Autodesk Inventor part; units mm, degrees
ref_plane "YZ Plane" through (0, 0, 0) normal (1, 0, 0) x (0, 1, 0)
ref_plane "XZ Plane" through (0, 0, 0) normal (0, 1, 0) x (-1, 0, 0)
ref_plane "XY Plane" through (0, 0, 0) normal (0, 0, 1) x (1, 0, 0)
ref_plane "Work Plane1" through (32.4858, 0, 0) normal (0, 0, 1) x (1, 0, 0)
sketch "Sketch1" plane through (32.4858, 0, 0) normal (0, 0, 1) x (1, 0, 0)
  line L0 (-82.3611, -0.4) -> (-82.3611, 2.4)
  line L1 (-32.4858, 2) -> (-181.2976, 2)
  line L2 (-32.4858, 55) -> (-181.2976, 55)
  line L3 (-82.3611, 54.6) -> (-82.3611, 57.4)
  line L4 (-157.3611, 54.6) -> (-157.3611, 57.4)
  line L5 (-157.3611, -0.4) -> (-157.3611, 2.4)
  line L6 (-107.3611, -0.4) -> (-107.3611, 2.4)
  line L7 (-132.3611, -0.4) -> (-132.3611, 2.4)
  line L8 (-107.3611, 54.6) -> (-107.3611, 57.4)
  line L9 (-132.3611, 54.6) -> (-132.3611, 57.4)
  line L10 (-32.4858, 0) -> (-181.2976, 0)
  line L11 (-32.4858, 57) -> (-181.2976, 57)
  line L12 (-82.3611, 2) -> (-82.3611, 55) construction
  line L13 (-157.3611, 2) -> (-157.3611, 55) construction
  line L14 (-77.3611, 2) -> (-77.3611, 55)
  line L15 (-162.3611, 2) -> (-162.3611, 55)
  dimension "d0" = 5
  dimension "d1" = 5
ref_plane "Work Plane3" through (-129.8754, 2, 0) normal (1, 0, 0) x (0, 1, 0)
ref_plane "Work Plane2" through (1.0604, 0, 0) normal (0, 0, 1) x (-1, 0, 0)
sketch "Sketch2" plane through (-129.8754, 2, 0) normal (1, 0, 0) x (0, 1, 0)
  line L0 (0, 8.3309) -> (0, -17.2762)
  line L1 (53, 8.3309) -> (53, -17.2762)
  line L2 (53, -34) -> (55, -34)
  line L3 (53, -34) -> (55, -34)
  line L4 (-2, -34) -> (0, -34)
  line L5 (-2, -34) -> (0, -34)
  line L6 (53, -34) -> (0, -34) construction
  line L7 (53, -36) -> (0, -36)
  line L8 (0, 0) -> (53, 0) construction
  line L9 (0, 0) -> (0, -8) construction
  line L10 (53, 0) -> (53, -8) construction
  line L11 (47.871, -33) -> (5.129, -33)
  line L12 (53, -29) -> (0, -29) construction
  line L13 (53, 2) -> (0, 2)
  line L14 (47.871, -1) -> (5.129, -1)
  line L15 (53, -5) -> (0, -5) construction
  line L16 (5.129, -33) -> (26.5, -20.5)
  line L17 (32.4839, -17) -> (53, -5)
  line L18 (5.129, -1) -> (26.5, -13.5)
  line L19 (32.4839, -17) -> (53, -29)
  line L20 (0, -29) -> (20.5161, -17)
  line L21 (26.5, -13.5) -> (47.871, -1)
  line L22 (0, -5) -> (20.5161, -17)
  line L23 (26.5, -20.5) -> (47.871, -33)
  line L24 (53, 2) -> (53, -5)
  line L25 (0, 2) -> (0, -5)
  line L26 (0, -29) -> (0, -36)
  line L27 (53, -29) -> (53, -36)
  point P0 (-2, 0)
  dimension "d20" = 2
  dimension "d37" = 1
  dimension "d38" = 4
  dimension "d39" = 2
  dimension "d40" = 1
  dimension "d41" = 4
extrude "Extrusion2" add sketch "Sketch2" along normal blind 85
sketch "Sketch3" plane through (-129.8754, 55, -29) normal (0, 1, 0) x (1, 0, 0)
  line L0 (0, -12) -> (85, -12)
  point P0 (129.8754, -29)
sketch "Sketch4" plane through (-129.8754, 2, 0) normal (-1, 0, 0) x (0, 0, 1)
  line L0 (-13.5, 26.5) -> (-1, 47.871)
  line L1 (-1, 47.871) -> (-1, 5.129)
  line L2 (-1, 5.129) -> (-13.5, 26.5)
  line L3 (-20.5, 26.5) -> (-33, 5.129)
  line L4 (-33, 5.129) -> (-33, 47.871)
  line L5 (-33, 47.871) -> (-20.5, 26.5)
  line L6 (-36, 53) -> (-36, 0)
  line L7 (-36, 0) -> (-29, 0)
  line L8 (-29, 0) -> (-17, 20.5161)
  line L9 (-17, 20.5161) -> (-5, 0)
  line L10 (-5, 0) -> (2, 0)
  line L11 (2, 0) -> (2, 53)
  line L12 (2, 53) -> (-5, 53)
  line L13 (-5, 53) -> (-17, 32.4839)
  line L14 (-17, 32.4839) -> (-29, 53)
  line L15 (-29, 53) -> (-36, 53)
  point P0 (0, -2)
extrude "Extrusion3" cut sketch "Sketch4" against normal blind 25
properties part number "legspacer_paula"
Source: CAD feature listing. Evaluate the final solid. Frame: model axes, mm. A direction names the side the tool comes from. Give positions to 0.01 mm unless a question says otherwise; leave off trailing zeros. Write each loop counter-clockwise with the first axis right and the second up, starting at its lowest first coordinate (ties: lowest second). Pieces come first, ordered by that corner, then holes. Notation, with made-up numbers: (-20.5, 78.5) -> (12.5, 78.5) arc R23 ccw to (12.5, 93.5) -> close; hole circle Ø4 at (0.5, -0.75). An arc over 180 degrees is marked (long way). Write item = value, one per line.
Q1. Cut plane A-A on x = -71.5. Return loops of the section in (y, z), then the cut area to 3 significant figures.
Here are the results:
outline = (2, -36) -> (55, -36) -> (55, -29) -> (34.48, -17) -> (55, -5) -> (55, 2) -> (2, 2) -> (2, -5) -> (22.52, -17) -> (2, -29) -> close; hole (7.13, -33) -> (49.87, -33) -> (28.5, -20.5) -> close; hole (7.13, -1) -> (28.5, -13.5) -> (49.87, -1) -> close
area = 987 mm²
Q2. Cut plane D-D on y = 51. Return loops of the section in (x, z), then the cut area to 3 significant figures.
Here are the results:
outline = (-104.88, -36) -> (-44.88, -36) -> (-44.88, -26.66) -> (-104.88, -26.66) -> close; (-104.88, -7.34) -> (-44.88, -7.34) -> (-44.88, 2) -> (-104.88, 2) -> close
area = 1,120 mm²
Q3. Cut plane C-C on z = -7. Return loops of the section in (x, y), then the cut area to 3 significant figures.
Here are the results:
outline = (-104.88, 5.42) -> (-44.88, 5.42) -> (-44.88, 17.39) -> (-104.88, 17.39) -> close; (-104.88, 39.61) -> (-44.88, 39.61) -> (-44.88, 51.58) -> (-104.88, 51.58) -> close
area = 1,440 mm²
Q4. Mould query, pull axis Z, two halves, no side actions, for faces 1 (the face through (-75, 2, -1)), 2 (the face through (-75.295, 39.036, -7.338)), 3 (the face through (-75, 29, -36)). Classes: +Z half, -Z half, draft (parallel to the pull), parting line (faces both ways), or undercut.
Here are the results:
face_1 = draft
face_2 = undercut
face_3 = -Z half
Q5. First-contact query: pin 1 (1.5 mm diameter, centred on x = -63, z = -23, fed in from +Y); pin 2 (6 mm diameter, centred on x = -62, z = -16, fed in from +Y). Flat tips, straight axial feed; report the tip coordinate or a pass-through.
Here are the results:
pin_1 = 46.02
pin_2 = 41.32
Q6. Cut plane B-B on y = 23.5. Return loops of the section in (x, z).
Here are the results:
outline = (-104.88, -36) -> (-44.88, -36) -> (-44.88, -33) -> (-104.88, -33) -> close; (-104.88, -23.42) -> (-44.88, -23.42) -> (-44.88, -10.58) -> (-104.88, -10.58) -> close; (-104.88, -1) -> (-44.88, -1) -> (-44.88, 2) -> (-104.88, 2) -> close
Q7. Line query: line 1 (Z direction, x = -82, y = 21.5); line 2 (Z direction, x = -64, y = 19); line 3 (Z direction, x = -81.5, y = 33.5). Output: solid intervals per line, ascending. Write a range as from..to.
Here are the results:
line_1 = -36..-33, -24.59..-17.59, -16.41..-9.41, -1..2
line_2 = -36..-33, -26.06..-19.06, -14.94..-7.94, -1..2
line_3 = -36..-33, -23.42..-10.58, -1..2
Q8. Reachability of faces 4 (the face through (-75, 55, -32)), 5 (the face through (-75.295, 44.598, -11.084)), 6 (the face through (-75, 2, -32)), 7 (the face through (-75, 29, -33)), 8 (the face through (-75.295, 12.114, -23.084)) from +Z, -Z, +X, -X, +Y, -Y: full face, straight path, thin tool, end or side. Return the list, or none.
Here are the results:
face_4 = +Z, -Z, +X, -X, +Y
face_5 = +X, -X, +Y
face_6 = +Z, -Z, +X, -X, -Y
face_7 = +X, -X
face_8 = +X, -X, -Y
